Verification items for the finished model (mm, model axes). Face numbers are marked on the shaded views. A direction names the side the tool comes from. Coordinates: 2 decimals unless noted, no trailing zeros. Order: outer loops, then holes, each group sorted by start corner. A loop starts at its lowest first (then second) coordinate and runs counter-clockwise, first axis right, second up.
Q1. Cross-section at C-C, the plane z = -1. Record the boundary of the cut face in (x, y).
Q2. Cross-section at B-B, the plane y = -8. Record the boundary of the cut face in (x, z).
Q3. Cross-section at A-A, the plane x = 15. Record the boundary of the cut face in (y, z), and give its area (3 significant figures).
Q4. Cross-section at D-D, the plane z = 20. Record the boundary of the cut face in (x, y).
Q5. Set-up check for the marked faces 1, 2, 3 and 4: record each of +Z, -Z, +X, -X, +Y, -Y from which the full face is reachable in a straight line by a thin tool's end or side.
Q6. Thickness scan on line 1 (X direction, y = -11.5, z = 6); line 2 (Z direction, x = 13, y = -16); line 3 (Y direction, x = 7.5, z = 13). Record the ranges inside material, lowest first.
Q7. Depth check by flat-ended pin: P1, Ø0.9, axis at y = 5.5, z = 11.5, coming from the -X side; P2, Ø10, axis at y = -13.5, z = 18.5, coming from the -X side; P3, Ø3.5, axis at x = -15, y = -4.37, coming from the +Z side; P4, Ø17, axis at x = 1.5, z = 22.5, coming from the +Y side. Enter the tip coordinate at first touch or a pass-through.
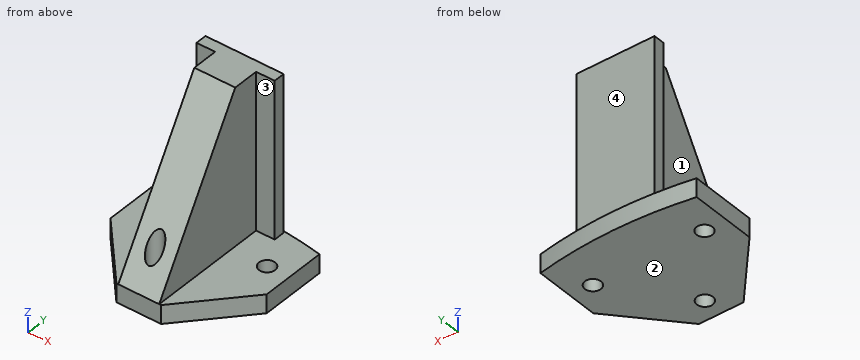
from build123d import *

# Parameters (mm, degrees)
BOSS_EXTRUDE1_DEPTH      = 42
BOSS_EXTRUDE3_DEPTH      = 5
SKETCH5_R                = 2.15
CUT_EXTRUDE4_DEPTH       = 5
BOSS_EXTRUDE4_DEPTH      = 8
BOSS_EXTRUDE4_DEPTH_BACK = 8
ENL_V_START              = -42
ESQUISSE2_W              = 18.319626144
ESQUISSE2_H              = 0.2
ENL_V_MAT_EXTRU_1_DEPTH  = 42
ESQUISSE4_W              = 42
ESQUISSE4_H              = 5
BOSS_EXTRU_2_DEPTH       = 15
ESQUISSE5_R              = 2.15
ENL_V_MAT_EXTRU_2_DEPTH  = 28
ENL_V_START_2            = -5
ENL_V_MAT_EXTRU_3_DEPTH  = 5
BOSS_EXTRU_3_DEPTH       = 5.8
BOSS_EXTRU_4_DEPTH       = 15
ESQUISSE14_W             = 44.082286315
ESQUISSE14_H             = 62.535336401
ENL_V_MAT_EXTRU_4_DEPTH  = 50
BOSS_EXTRU_5_DEPTH       = 42
BOSS_EXTRU_7_DEPTH       = 11
ESQUISSE20_R             = 2.15
ENL_V_MAT_EXTRU_7_DEPTH  = 42
BOSS_EXTRU_8_START       = -5
BOSS_EXTRU_8_DEPTH       = 5


# Read off the part's stored shape, not the designer's step: Enlèv. mat.-Extru.3
with BuildPart() as part:
    # Sketch1 → Boss-Extrude1 (new body)
    with BuildSketch(Plane.XY):
        Polygon((-8.8, 3), (-6.002154051, -3), (6.002154051, -3), (8.8, 3), align=None)
    extrude(amount=BOSS_EXTRUDE1_DEPTH)

    # Sketch2 → Boss-Extrude3 (add)
    with BuildSketch(Plane(origin=(0, 0, 0), x_dir=(-1, 0, 0), z_dir=(0, 0, -1))):
        with BuildLine():
            Line((21, 4.736174234), (21, -13.75))
            Line((21, -13.75), (-21, -13.75))
            Line((-21, -13.75), (-21, 4.736174234))
            ThreePointArc((-21, 4.736174234), (0, 6.759324864), (21, 4.736174234))
        make_face()
    extrude(amount=BOSS_EXTRUDE3_DEPTH)

    # Sketch5 → Cut-Extrude4 (cut)
    with BuildSketch(Plane(origin=(0, 0, -5), x_dir=(-1, 0, 0), z_dir=(0, 0, -1))):
        with Locations((-15, -4.37207547)):
            Circle(SKETCH5_R)
        with Locations((15, -4.37207547)):
            Circle(SKETCH5_R)
    extrude(amount=-CUT_EXTRUDE4_DEPTH, mode=Mode.SUBTRACT)

    # Sketch4 → Boss-Extrude4 (add, two sides: drawn at the far end of the back side and taken through both)
    with BuildSketch(Plane.ZY.offset(-BOSS_EXTRUDE4_DEPTH_BACK)):
        Polygon((42, -3), (0, -3), (0, -26), (15, -26), (15, -17.785714286), align=None)
    extrude(amount=BOSS_EXTRUDE4_DEPTH + BOSS_EXTRUDE4_DEPTH_BACK)

    # Esquisse2 → Enlèv. mat.-Extru.1 (cut)
    with BuildSketch(Plane.XY.offset(42).offset(ENL_V_START)):
        with Locations((-0.359813072, 2.9)):
            Rectangle(ESQUISSE2_W, ESQUISSE2_H)
    extrude(amount=ENL_V_MAT_EXTRU_1_DEPTH, mode=Mode.SUBTRACT)

    # Esquisse4 → Boss.-Extru.2 (add)
    with BuildSketch(Plane.XZ.offset(13.75)):
        with Locations((0, -2.5)):
            Rectangle(ESQUISSE4_W, ESQUISSE4_H)
    extrude(amount=BOSS_EXTRU_2_DEPTH)

    # Esquisse5 → Enlèv. mat.-Extru.2 (cut)
    with BuildSketch(Plane(origin=(0, 0, -5), x_dir=(-1, 0, 0), z_dir=(0, 0, -1))):
        with Locations((0, -23.240675136)):
            Circle(ESQUISSE5_R)
    extrude(amount=-ENL_V_MAT_EXTRU_2_DEPTH, mode=Mode.SUBTRACT)

    # Enlèv. mat.-Extru.3 outline → Enlèv. mat.-Extru.3 (cut)
    with BuildSketch(Plane(origin=(0, 0, -5), x_dir=(-1, 0, 0), z_dir=(0, 0, -1)).offset(ENL_V_START_2)):
        Polygon((21, -12.006912883), (6, -28.75), (21, -28.75), align=None)
        Polygon((-6, -28.75), (-21, -12.006912883), (-21, -28.75), align=None)
    extrude(amount=ENL_V_MAT_EXTRU_3_DEPTH, mode=Mode.SUBTRACT)

    # Esquisse7 → Boss.-Extru.3 (add)
    with BuildSketch(Plane(origin=(0, 2.8, 0), x_dir=(1, 0, 0), z_dir=(0, 1, 0))):
        with BuildLine():
            Line((2.5, -42), (0, -42))
            Line((0, -42), (-2.5, -42))
            Line((-2.5, -42), (-2.5, -42.178964355))
            ThreePointArc((-2.5, -42.178964355), (0, -47.633030278), (2.5, -42.178964355))
            Line((2.5, -42.178964355), (2.5, -42))
        make_face()
    extrude(amount=-BOSS_EXTRU_3_DEPTH)

    # Esquisse9 → Boss.-Extru.4 (add)
    with BuildSketch(Plane.XY):
        Polygon((8, -26), (8, -26.146615259), (6, -28.75), (-6, -28.75), (-8, -26.360097245), (-8, -26), align=None)
    extrude(amount=BOSS_EXTRU_4_DEPTH)

    # Esquisse14 → Enlèv. mat.-Extru.4 (cut)
    with BuildSketch(Plane.XY):
        with Locations((2.134773814, -3.901083115)):
            Rectangle(ESQUISSE14_W, ESQUISSE14_H)
    extrude(amount=ENL_V_MAT_EXTRU_4_DEPTH, mode=Mode.SUBTRACT)

    # Esquisse15 → Boss.-Extru.5 (add)
    with BuildSketch(Plane.XY):
        Polygon((-10.5, 6.8), (10.5, 6.8), (10.5, 3.8), (5.5, 3.8), (5.5, -3.2), (-5.5, -3.2), (-5.5, 3.8), (-10.5, 3.8), align=None)
    extrude(amount=BOSS_EXTRU_5_DEPTH)

    # Esquisse16 → Boss.-Extru.7 (add)
    with BuildSketch(Plane(origin=(5.5, 0, 0), x_dir=(0, 0, -1), z_dir=(1, 0, 0))):
        Polygon((0, -3.2), (0, -28.75), (-42, -3.2), align=None)
    extrude(amount=-BOSS_EXTRU_7_DEPTH)

    # Esquisse20 → Enlèv. mat.-Extru.7 (cut)
    with BuildSketch(Plane(origin=(0, 0, 0), x_dir=(-1, 0, 0), z_dir=(0, 0, -1))):
        with Locations((0, -23.240675136)):
            Circle(ESQUISSE20_R)
    extrude(amount=-ENL_V_MAT_EXTRU_7_DEPTH, mode=Mode.SUBTRACT)

    # Esquisse21 → Boss.-Extru.8 (add)
    with BuildSketch(Plane(origin=(0, 0, -5), x_dir=(-1, 0, 0), z_dir=(0, 0, -1)).offset(BOSS_EXTRU_8_START)):
        with BuildLine():
            Line((-21, 4.736174234), (-21, 5.754737611))
            ThreePointArc((-21, 5.754737611), (0, 7.759324864), (21, 5.754737611))
            Line((21, 5.754737611), (21, 4.736174234))
            ThreePointArc((21, 4.736174234), (0, 6.759324864), (-21, 4.736174234))
        make_face()
    extrude(amount=BOSS_EXTRU_8_DEPTH)


solid = part.part
Check values:
1. outline: (-21, -12.01) - (-6, -28.75) - (6, -28.75) - (21, -12.01) - (21, 5.75) arc R111 ccw to (-21, 5.75) - close; hole circle Ø4.3 at (-15, -4.37); hole circle Ø4.3 at (0, -23.24); hole circle Ø4.3 at (15, -4.37)
2. outline: (-21, -5) - (21, -5) - (21, 0) - (5.5, 0) - (5.5, 34.11) - (-5.5, 34.11) - (-5.5, 0) - (-21, 0) - close
3. outline: (-18.7, -5) - (-6.52, -5) - (-6.52, 0) - (-18.7, 0) - close; (-2.22, -5) - (6.74, -5) - (6.74, 0) - (-2.22, 0) - close
3. area: 106 mm2
4. outline: (-10.5, 3.8) - (-5.5, 3.8) - (-5.5, -16.58) - (5.5, -16.58) - (5.5, 3.8) - (10.5, 3.8) - (10.5, 6.8) - (-10.5, 6.8) - close
5. face 1: +Z, -X, -Y
5. face 2: -Z, +X, -X, +Y, -Y
5. face 3: +Z, +X, -Y
5. face 4: +Z, +X, -X, +Y
6. line 1: x = -5.5 to 5.5
6. line 2: z = -5 to 0
6. line 3: y = 3.8 to 6.8
7. P1: stops at x = -10.5
7. P2: stops at x = -5.5
7. P3: passes through
7. P4: stops at y = 6.8
